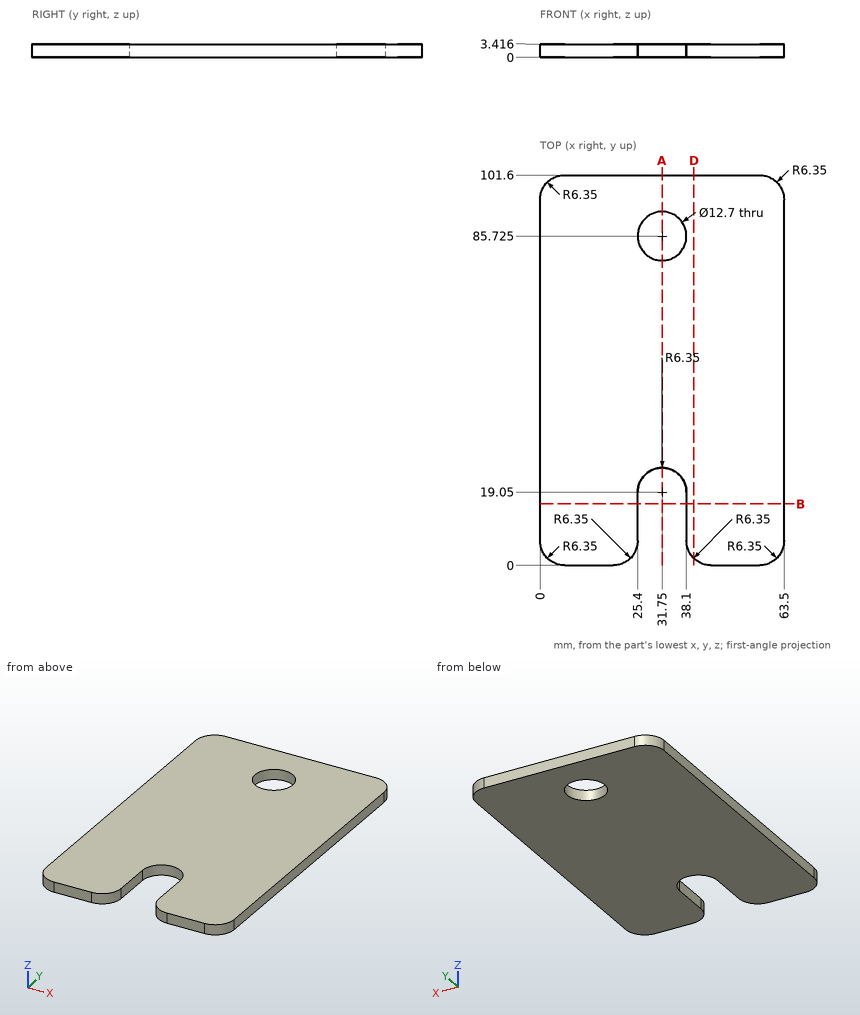
For this review, use the dimensioned drawing (mm, ordinates from the lowest corner) and the shaded views. Round coordinates to 2 decimals unless told otherwise and drop trailing zeros. Order: outer loops, then holes, each group sorted by start corner. A loop starts at its lowest first (then second) coordinate and runs counter-clockwise, first axis right, second up. Notation, with made-up numbers: (37, -6) - (72, -6) arc R15 cw to (72, 20) - close; hole circle Ø5 at (-3.5, 78.25). An arc over 180 degrees is marked (long way). Use one line per item in the form item = value.
Q1. To check wall thickness, follow line 1 (Y direction, x = 31.75, z = 1.1) (1 decimal); line 2 (X direction, y = 4.5, z = 0.4) (1 decimal); line 3 (Y direction, x = 6, z = 2.2). State the ranges of each line that lie inside material, in increasing order.
Response values:
line_1 = 25.4 to 79.4, 92.1 to 101.6
line_2 = 0.3 to 25.1, 38.4 to 63.2
line_3 = 0.01 to 101.59
Q2. Add section D-D on x = 40. Give the boundary of the cut face in (y, z).
Response values:
outline = (1.82, 0) - (101.6, 0) - (101.6, 3.42) - (1.82, 3.42) - close
Q3. Add section B-B on y = 16. Give the boundary of the cut face in (x, z).
Response values:
outline = (0, 0) - (25.4, 0) - (25.4, 3.42) - (0, 3.42) - close; (38.1, 0) - (63.5, 0) - (63.5, 3.42) - (38.1, 3.42) - close
Q4. Add section A-A on x = 31.75. Give the boundary of the cut face in (y, z) (1 decimal).
Response values:
outline = (25.4, 0) - (79.4, 0) - (79.4, 3.4) - (25.4, 3.4) - close; (92.1, 0) - (101.6, 0) - (101.6, 3.4) - (92.1, 3.4) - close
